Check sheet for the drawn part. Datum: minimum x, y, z corner. Units: mm. A direction names the side the tool comes from. Round coordinates to 2 decimals unless told otherwise and drop trailing zeros. Write each loop counter-clockwise with the first axis right and the second up, starting at its lowest first coordinate (ties: lowest second). Pieces come first, ordered by that corner, then holes. Notation, with made-up numbers: (56, -12.5) - (62, -12.5) arc R13 ccw to (62, -6.5) - close; hole circle Ø1 at (43, -38.5). An arc over 180 degrees is marked (long way). Answer as a JSON object with one key per item and string values. Group by question number.
Item 1: Set-up check for the marked faces 1 and 2: record each of +Z, -Z, +X, -X, +Y, -Y from which the full face is reachable in a straight line by a thin tool's end or side.
Item 2: Gauge pin test, flat ends, axial feed: P1, Ø1.5, axis at y = 16.5, z = 2.5, coming from the -X side; P2, Ø1.5, axis at x = 12.5, z = 2, coming from the +Y side; P3, Ø4.5, axis at x = 60, y = 9.75, coming from the -Z side. Record the tip position at first contact, or that the pin passes through.
Item 3: Sectioned sample at D-D on y = 15.5. Record the boundary of the cut face in (x, z).
Item 4: Thickness scan on line 1 (X direction, y = 9.75, z = 1.85); line 2 (Y direction, x = 60, z = 3.45); line 3 (Y direction, x = 43.5, z = 3.6). Record the ranges inside material, lowest first.
Item 5: Sectioned sample at B-B on y = 9.75. Record the boundary of the cut face in (x, z), plus the area to 3 significant figures.
Item 6: Sectioned sample at C-C on z = 4.3. Record the boundary of the cut face in (x, y), plus the area to 3 significant figures.
Item 7: Sectioned sample at A-A on x = 60. Record the boundary of the cut face in (y, z), plus the area to 3 significant figures.
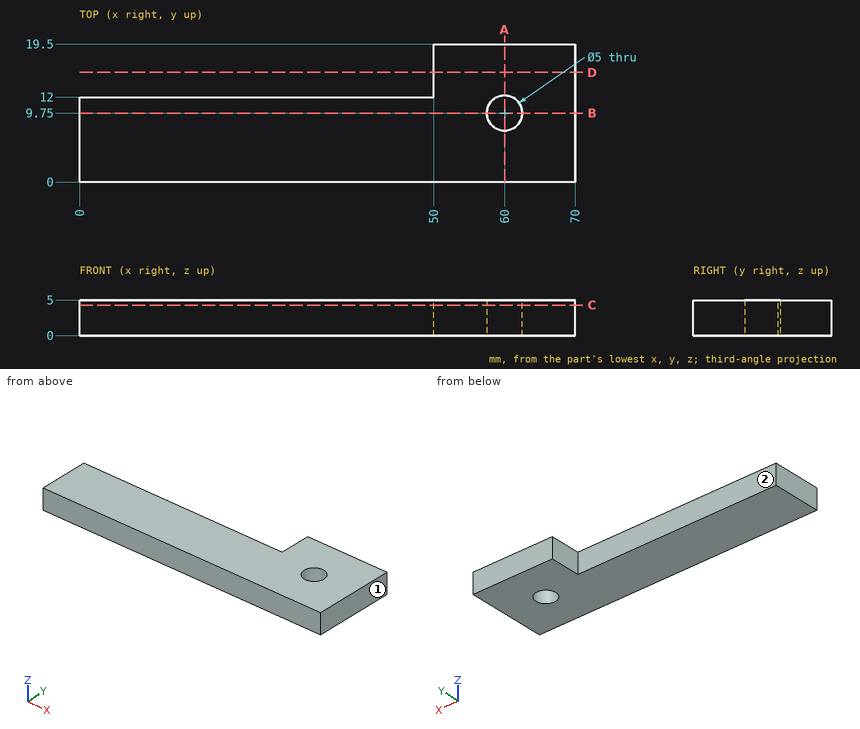
Completed:
{
 "1": {"face 1": "+Z, -Z, +X, +Y, -Y", "face 2": "+Z, -Z, -X, +Y"},
 "2": {"P1": "x = 50", "P2": "y = 12", "P3": "through"},
 "3": {"outline": "(50, 0) - (70, 0) - (70, 5) - (50, 5) - close"},
 "4": {"line 1": "0 to 57.5, 62.5 to 70", "line 2": "0 to 7.25, 12.25 to 19.5", "line 3": "0 to 12"},
 "5": {"outline": "(0, 0) - (57.5, 0) - (57.5, 5) - (0, 5) - close; (62.5, 0) - (70, 0) - (70, 5) - (62.5, 5) - close", "area": "325 mm²"},
 "6": {"outline": "(0, 0) - (70, 0) - (70, 19.5) - (50, 19.5) - (50, 12) - (0, 12) - close; hole circle Ø5 at (60, 9.75)", "area": "970 mm²"},
 "7": {"outline": "(0, 0) - (7.25, 0) - (7.25, 5) - (0, 5) - close; (12.25, 0) - (19.5, 0) - (19.5, 5) - (12.25, 5) - close", "area": "72.5 mm²"}
}
